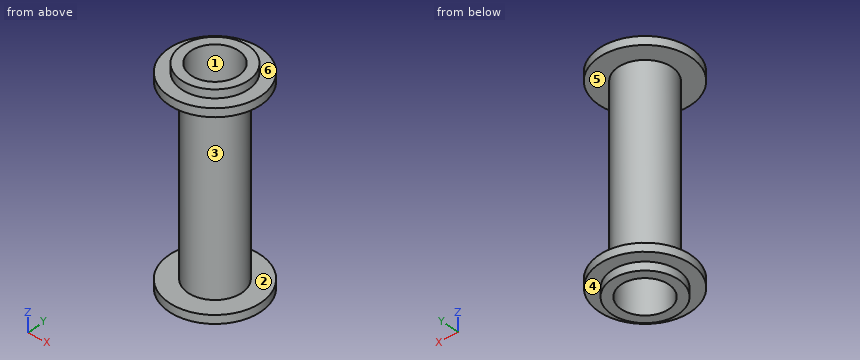
```python
from build123d import *

# Parameters (mm, degrees)
SKETCH1_R           = 8
BOSS_EXTRUDE1_DEPTH = 2
SKETCH2_R           = 11
BOSS_EXTRUDE2_DEPTH = 2
SKETCH3_R           = 6.45
BOSS_EXTRUDE3_DEPTH = 44
SKETCH4_R           = 11
BOSS_EXTRUDE4_DEPTH = 2
SKETCH5_R           = 8
BOSS_EXTRUDE5_DEPTH = 2
SKETCH6_R           = 5.7
CUT_EXTRUDE1_DEPTH  = 53


with BuildPart() as part:
    # Sketch1 → Boss-Extrude1 (new body)
    with BuildSketch(Plane.XY):
        Circle(SKETCH1_R)
    extrude(amount=BOSS_EXTRUDE1_DEPTH)

    # Sketch2 → Boss-Extrude2 (add)
    with BuildSketch(Plane.XY.offset(2)):
        Circle(SKETCH2_R)
    extrude(amount=BOSS_EXTRUDE2_DEPTH)

    # Sketch3 → Boss-Extrude3 (add)
    with BuildSketch(Plane.XY.offset(4)):
        Circle(SKETCH3_R)
    extrude(amount=BOSS_EXTRUDE3_DEPTH)

    # Sketch4 → Boss-Extrude4 (add)
    with BuildSketch(Plane.XY.offset(48)):
        Circle(SKETCH4_R)
    extrude(amount=BOSS_EXTRUDE4_DEPTH)

    # Sketch5 → Boss-Extrude5 (add)
    with BuildSketch(Plane.XY.offset(50)):
        Circle(SKETCH5_R)
    extrude(amount=BOSS_EXTRUDE5_DEPTH)

    # Sketch6 → Cut-Extrude1 (cut, through all)
    with BuildSketch(Plane.XY.offset(52)):
        Circle(SKETCH6_R)
    extrude(amount=-CUT_EXTRUDE1_DEPTH, mode=Mode.SUBTRACT)


solid = part.part
```
Build history of the part. All positions in model axes, mm. Face numbers are marked on the shaded views. A direction names the side the tool comes from. Give positions to 0.01 mm unless a question says otherwise; leave off trailing zeros. Loops run counter-clockwise (first coordinate to the right, second up) from the corner with the lowest first, then second, coordinate; pieces in that order, holes last. Notation, with made-up numbers: (-12, 85.25) - (14, 85.25) arc R30 ccw to (14, 117.25) - close; hole circle Ø8 at (-26, 83). An arc over 180 degrees is marked (long way). Use a Markdown table: item, result.
(1) Pull direction X, two halves, no side cores. Call the marked faces 1, 2 and 3: +X half, -X half, draft (parallel to the pull), parting line (faces both ways), or undercut.
Taken from the geometry:
| item | result |
|---|---|
| face 1 | undercut |
| face 2 | draft |
| face 3 | parting line |
(2) Band-saw the part on A-A (x = 0). Give the cut face in (y, z).
Taken from the geometry:
| item | result |
|---|---|
| outline | (-11, 2) - (-8, 2) - (-8, 0) - (-5.7, 0) - (-5.7, 52) - (-8, 52) - (-8, 50) - (-11, 50) - (-11, 48) - (-6.45, 48) - (-6.45, 4) - (-11, 4) - close; (5.7, 0) - (8, 0) - (8, 2) - (11, 2) - (11, 4) - (6.45, 4) - (6.45, 48) - (11, 48) - (11, 50) - (8, 50) - (8, 52) - (5.7, 52) - close |
(3) Drop flat-ended pins along their axis: pin 1 Ø10 at (x, z) = (-0.5, 41.5) entering from +Y; pin 2 Ø12 at (y, z) = (-4.5, 40) entering from +X; pin 3 Ø3 at (x, y) = (8, 3.5) entering from -Z; pin 4 Ø3 at (x, z) = (-6, 7) entering from -Y. Give the stop position or say it passes through.
Taken from the geometry:
| item | result |
|---|---|
| pin 1 | y = 6.45 |
| pin 2 | x = 6.45 |
| pin 3 | z = 0 |
| pin 4 | y = -4.62 |
(4) Band-saw the part on D-D (y = -8.5). Give the cut face in (x, z), and give its area (3 significant figures).
Taken from the geometry:
| item | result |
|---|---|
| outline | (-6.98, 2) - (6.98, 2) - (6.98, 4) - (-6.98, 4) - close; (-6.98, 48) - (6.98, 48) - (6.98, 50) - (-6.98, 50) - close |
| area | 55.9 mm2 |
(5) Band-saw the part on C-C (z = 42.5). Give the cut face in (x, y).
Taken from the geometry:
| item | result |
|---|---|
| outline | circle Ø12.9 at (0, 0); hole circle Ø11.4 at (0, 0) |
(6) Which spindle directions (+Z, -Z, +X, -X, +Y, -Y) get a long thin tool onto all of the face, cutting with end or side? Do the marked faces 4, 5 and 6. Say none if no direction does.
Taken from the geometry:
| item | result |
|---|---|
| face 4 | -Z |
| face 5 | none |
| face 6 | +Z |
(7) Wall check: line 1 along Z through (x, y) = (10, -0.75); line 2 along Y through (x, z) = (0, 36); line 3 along Z through (x, y) = (1.5, -7). Give the ranges that are in metal, low to high.
Taken from the geometry:
| item | result |
|---|---|
| line 1 | 2 to 4, 48 to 50 |
| line 2 | -6.45 to -5.7, 5.7 to 6.45 |
| line 3 | 0 to 4, 48 to 52 |
